The listing builds one solid part. Answer for the finished solid, in the listing's coordinates (mm). Face numbers are marked on the shaded views. A direction names the side the tool comes from. Give positions to 0.01 mm unless a question says otherwise; leave off trailing zeros. Order: outer loops, then holes, each group sorted by start corner. A loop starts at its lowest first (then second) coordinate and runs counter-clockwise, first axis right, second up. Notation, with made-up numbers: (-30.75, -4.75) - (23.25, -4.75) arc R23 ccw to (23.25, 11.25) - close; hole circle Ø7 at (-35, 16). An arc over 180 degrees is marked (long way). Use a Markdown table: item, result. Add a question column.
1) Find section C-C, the plane x = 5. Determine the outline of the cut face in (y, z) (3 decimals), plus the area to 3 significant figures.
2) For the marked faces 1 and 2, determine the directions among +Z, -Z, +X, -X, +Y, -Y from which every point of the face is accessible in a straight line to the end or side of a thin tool.
3) Find section B-B, the plane z = 18. Determine the outline of the cut face in (x, y) (3 decimals), plus the area to 3 significant figures.
4) Straight lines are drawn through the part: line 1 (Z direction, x = -18, y = -6); line 2 (Y direction, x = 8, z = 14); line 3 (Z direction, x = -3, y = 30). For each, find the intervals that lie inside material, in ascending order.
5) Find section A-A, the plane y = 0. Determine the outline of the cut face in (x, z) (3 decimals), plus the area to 3 significant figures.
6) Find section D-D, the plane y = 29.5. Determine the outline of the cut face in (x, z), plus the area to 3 significant figures.
7) Flat-ended cylindrical pins translate along their axes: pin 1 (3 mm diameter, centred on x = -5.5, y = 11, fed in from +Z) (3 decimals); pin 2 (4 mm diameter, centred on x = -3.5, z = 23, fed in from +Y); pin 3 (0.9 mm diameter, centred on x = -15.5, y = 15, fed in from +Z); pin 4 (24 mm diameter, centred on x = -3, y = -0.5, fed in from +Z). Find the tip coordinate at first contact, or state that the pin passes through.
from build123d import *

# Parameters (mm, degrees)
SKETCH1_W           = 40.132
SKETCH1_H           = 40.132
BOSS_EXTRUDE1_DEPTH = 22.7584
SKETCH2_W           = 0.4826
SKETCH2_H           = 92.619583511
SKETCH3_W           = 0.4826
SKETCH3_H           = 92.619583511
SKETCH4_W           = 0.4826
SKETCH4_H           = 92.619583511
SKETCH5_W           = 0.4826
SKETCH5_H           = 92.619583511
HOLE1_D             = 2.8448
HOLE1_DEPTH         = 21.9964
HOLE2_D             = 2.8448
HOLE2_DEPTH         = 21.9964
HOLE3_D             = 2.8448
HOLE3_DEPTH         = 21.9964
HOLE4_D             = 2.8448
HOLE4_DEPTH         = 21.9964
FILLET1_R           = 3.175
FILLET2_R           = 3.175
FILLET3_R           = 3.175
FILLET4_R           = 3.175


with BuildPart() as part:
    # Sketch1 → Boss-Extrude1 (new body)
    with BuildSketch(Plane.XY.offset(22.7584)):
        Rectangle(SKETCH1_W, SKETCH1_H)
    extrude(amount=-BOSS_EXTRUDE1_DEPTH)

    # Sketch2 → Revolve1 (revolve)
    with BuildSketch(Plane(origin=(0, 0, 2.2098), x_dir=(-1, 0, 0), z_dir=(0, 0, -1))):
        with Locations((2.8067, 66.375791756)):
            Rectangle(SKETCH2_W, SKETCH2_H)
    revolve(axis=Axis((-3.048, 20.066, 2.2098), (0, 1, 0)))

    # Sketch3 → Revolve2 (revolve)
    with BuildSketch(Plane(origin=(0, 0, 2.2098), x_dir=(-1, 0, 0), z_dir=(0, 0, -1))):
        with Locations((-1.2573, 66.375791756)):
            Rectangle(SKETCH3_W, SKETCH3_H)
    revolve(axis=Axis((1.016, 20.066, 2.2098), (0, 1, 0)))

    # Sketch4 → Revolve3 (revolve)
    with BuildSketch(Plane(origin=(0, 0, 2.2098), x_dir=(-1, 0, 0), z_dir=(0, 0, -1))):
        with Locations((-3.2893, 66.375791756)):
            Rectangle(SKETCH4_W, SKETCH4_H)
    revolve(axis=Axis((3.048, 20.066, 2.2098), (0, 1, 0)))

    # Sketch5 → Revolve4 (revolve)
    with BuildSketch(Plane(origin=(0, 0, 2.2098), x_dir=(-1, 0, 0), z_dir=(0, 0, -1))):
        with Locations((0.7747, 66.375791756)):
            Rectangle(SKETCH5_W, SKETCH5_H)
    revolve(axis=Axis((-1.016, 20.066, 2.2098), (0, 1, 0)))

    # Sketch6 → Revolve5 (revolve)
    with BuildSketch(Plane(origin=(0, 0, 0), x_dir=(1, 0, 0), z_dir=(0, 1, 0))):
        Polygon((10.9982, -22.7584), (0, -22.7584), (0, -37.9984), (2.49936, -37.9984), (2.49936, -24.765), (10.9982, -24.765), align=None)
    revolve(axis=Axis((0, 0, 22.7584), (0, 0, 1)))

    # Hole1
    with Locations(Plane.XY.offset(22.7584)):
        with Locations((-15.494, 15.494)):
            Hole(HOLE1_D / 2, depth=HOLE1_DEPTH)

    # Hole2
    with Locations(Plane.XY.offset(22.7584)):
        with Locations((15.494, 15.494)):
            Hole(HOLE2_D / 2, depth=HOLE2_DEPTH)

    # Hole3
    with Locations(Plane.XY.offset(22.7584)):
        with Locations((-15.494, -15.494)):
            Hole(HOLE3_D / 2, depth=HOLE3_DEPTH)

    # Hole4
    with Locations(Plane.XY.offset(22.7584)):
        with Locations((15.494, -15.494)):
            Hole(HOLE4_D / 2, depth=HOLE4_DEPTH)

    # Fillet1
    fillet1_edges = [part.edges().sort_by_distance(p)[0] for p in [
        (20.066, -20.066, 11.3792),
    ]]
    fillet(fillet1_edges, radius=FILLET1_R)

    # Fillet2
    fillet2_edges = [part.edges().sort_by_distance(p)[0] for p in [
        (-20.066, -20.066, 11.3792),
    ]]
    fillet(fillet2_edges, radius=FILLET2_R)

    # Fillet3
    fillet3_edges = [part.edges().sort_by_distance(p)[0] for p in [
        (20.066, 20.066, 11.3792),
    ]]
    fillet(fillet3_edges, radius=FILLET3_R)

    # Fillet4
    fillet4_edges = [part.edges().sort_by_distance(p)[0] for p in [
        (-20.066, 20.066, 11.3792),
    ]]
    fillet(fillet4_edges, radius=FILLET4_R)


solid = part.part
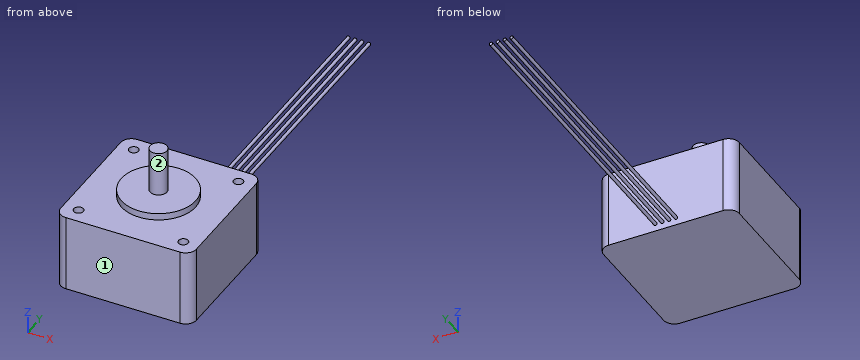
The answers:
| question | item | result |
|---|---|---|
| 1 | outline | (-20.066, 0) - (20.066, 0) - (20.066, 22.758) - (9.796, 22.758) - (9.796, 24.765) - (-9.796, 24.765) - (-9.796, 22.758) - (-20.066, 22.758) - close |
| 1 | area | 953 mm2 |
| 2 | face 1 | +Z, -Z, +X, -X, -Y |
| 2 | face 2 | +Z |
| 3 | outline | (-20.066, -16.891) arc R3.175 ccw to (-16.891, -20.066) - (16.891, -20.066) arc R3.175 ccw to (20.066, -16.891) - (20.066, 16.891) arc R3.175 ccw to (16.891, 20.066) - (-16.891, 20.066) arc R3.175 ccw to (-20.066, 16.891) - close; hole circle Ø2.845 at (-15.494, -15.494); hole circle Ø2.845 at (-15.494, 15.494); hole circle Ø2.845 at (15.494, -15.494); hole circle Ø2.845 at (15.494, 15.494) |
| 3 | area | 1,580 mm2 |
| 4 | line 1 | 0 to 22.76 |
| 4 | line 2 | -20.07 to 20.07 |
| 4 | line 3 | 1.73 to 2.69 |
| 5 | outline | (-20.066, 0) - (20.066, 0) - (20.066, 22.758) - (10.998, 22.758) - (10.998, 24.765) - (2.499, 24.765) - (2.499, 37.998) - (-2.499, 37.998) - (-2.499, 24.765) - (-10.998, 24.765) - (-10.998, 22.758) - (-20.066, 22.758) - close |
| 5 | area | 1,020 mm2 |
| 6 | outline | circle Ø0.97 at (-3.05, 2.21); circle Ø0.97 at (-1.02, 2.21); circle Ø0.97 at (1.02, 2.21); circle Ø0.97 at (3.05, 2.21) |
| 6 | area | 2.93 mm2 |
| 7 | pin 1 | z = 24.765 |
| 7 | pin 2 | y = 20.07 |
| 7 | pin 3 | z = 0.76 |
| 7 | pin 4 | z = 38 |
